```python
from build123d import *

# Parameters (mm, degrees)
SALIENTE_EXTRUIR1_DEPTH = 233
VACIADO1_T              = -2
SALIENTE_EXTRUIR2_REACH = 250.108
CROQUIS3_R              = 3.999999999999999
CROQUIS3_R_2            = 4.000000000000005
CROQUIS3_R_3            = 4.000000000000013
CROQUIS3_R_4            = 4.000000000000007
CROQUIS3_R_5            = 4.000000000000002
CROQUIS3_R_6            = 4
CROQUIS4_R              = 1.5000000000000007
CROQUIS4_R_2            = 1.4999999999999973
CROQUIS4_R_3            = 1.5000000000000042
CROQUIS4_R_4            = 1.5000000000000024
CROQUIS4_R_5            = 1.5000000000000009
CORTAR_EXTRUIR1_DEPTH   = 10
CROQUIS5_R              = 1.7500000000000002
CROQUIS5_R_2            = 1.7499999999999893
CROQUIS5_R_3            = 1.7500000000000038
CROQUIS5_R_4            = 1.749999999999997
CROQUIS5_R_5            = 1.7499999999999987
CROQUIS5_R_6            = 1.7500000000000004
CORTAR_EXTRUIR2_DEPTH   = 5
CROQUIS6_R              = 2.0000000000000036
CROQUIS6_R_2            = 1.9999999999999967
CROQUIS6_R_3            = 1.99999999999999
CROQUIS6_R_4            = 2.000000000000003
CORTAR_EXTRUIR3_DEPTH   = 1
CORTAR_EXTRUIR4_DEPTH   = 2
REDONDEO1_R             = 1


with BuildPart() as part:
    # Croquis1 → Saliente-Extruir1 (new body)
    with BuildSketch(Plane.XY):
        Polygon((82.35016819503933, 0), (82.35016819503927, 5.229344564858981), (80.29329266619476, 28.7395394398242), (78.30090327001128, 28.565227954328893), (1.9923893961834915, 21.889098059858902), (-1.33e-15, 21.7147865743636), (1.899797656141601, 0), align=None)
    extrude(amount=SALIENTE_EXTRUIR1_DEPTH)

    # Vaciado1
    vaciado1_openings = [part.faces().sort_by_distance(p)[0] for p in [
        (40.146646333, 25.227163007, 116.5),
    ]]
    offset(amount=VACIADO1_T, openings=vaciado1_openings, kind=Kind.INTERSECTION)

    # Saliente-Extruir2: up to this plane
    saliente_extruir2_end = Plane(origin=(1.899797656141601, 2, 233), z_dir=(0, 1, 0))
    # Croquis3 → Saliente-Extruir2 (add, up to the surface)
    with BuildSketch(Plane(origin=(-0.9092222397584271, 10.392457755273615, 0), x_dir=(0.9961946980917462, 0.08715574274765005, 0), z_dir=(-0.08715574274765005, 0.9961946980917462, 0)), mode=Mode.PRIVATE) as saliente_extruir2_sk1:
        with Locations((23.14256835249537, -4.200000000000009)):
            Circle(CROQUIS3_R)
    saliente_extruir2_tool1 = split(extrude(saliente_extruir2_sk1.sketch, amount=-SALIENTE_EXTRUIR2_REACH, mode=Mode.PRIVATE), bisect_by=saliente_extruir2_end, keep=Keep.BOTH, mode=Mode.PRIVATE)
    add(saliente_extruir2_tool1.solids().sort_by_distance((22.145282, 12.409465, 4.2))[0])
    # Croquis3 → Saliente-Extruir2 (add, up to the surface)
    with BuildSketch(Plane(origin=(-0.9092222397584271, 10.392457755273615, 0), x_dir=(0.9961946980917462, 0.08715574274765005, 0), z_dir=(-0.08715574274765005, 0.9961946980917462, 0)), mode=Mode.PRIVATE) as saliente_extruir2_sk2:
        with Locations(Location((61.24256835249536, -21.250000000000004, 0), (0, 0, 180))):
            Circle(CROQUIS3_R_2)
    saliente_extruir2_tool2 = split(extrude(saliente_extruir2_sk2.sketch, amount=-SALIENTE_EXTRUIR2_REACH, mode=Mode.PRIVATE), bisect_by=saliente_extruir2_end, keep=Keep.BOTH, mode=Mode.PRIVATE)
    add(saliente_extruir2_tool2.solids().sort_by_distance((60.1003, 15.730099, 21.25))[0])
    # Croquis3 → Saliente-Extruir2 (add, up to the surface)
    with BuildSketch(Plane(origin=(-0.9092222397584271, 10.392457755273615, 0), x_dir=(0.9961946980917462, 0.08715574274765005, 0), z_dir=(-0.08715574274765005, 0.9961946980917462, 0)), mode=Mode.PRIVATE) as saliente_extruir2_sk3:
        with Locations(Location((42.19256835249537, -97.45, 0), (0, 0, 180))):
            Circle(CROQUIS3_R_3)
    saliente_extruir2_tool3 = split(extrude(saliente_extruir2_sk3.sketch, amount=-SALIENTE_EXTRUIR2_REACH, mode=Mode.PRIVATE), bisect_by=saliente_extruir2_end, keep=Keep.BOTH, mode=Mode.PRIVATE)
    add(saliente_extruir2_tool3.solids().sort_by_distance((41.122791, 14.069782, 97.45))[0])
    # Croquis3 → Saliente-Extruir2 (add, up to the surface)
    with BuildSketch(Plane(origin=(-0.9092222397584271, 10.392457755273615, 0), x_dir=(0.9961946980917462, 0.08715574274765005, 0), z_dir=(-0.08715574274765005, 0.9961946980917462, 0)), mode=Mode.PRIVATE) as saliente_extruir2_sk4:
        with Locations(Location((61.24256835249536, -116.5, 0), (0, 0, 180))):
            Circle(CROQUIS3_R_4)
    saliente_extruir2_tool4 = split(extrude(saliente_extruir2_sk4.sketch, amount=-SALIENTE_EXTRUIR2_REACH, mode=Mode.PRIVATE), bisect_by=saliente_extruir2_end, keep=Keep.BOTH, mode=Mode.PRIVATE)
    add(saliente_extruir2_tool4.solids().sort_by_distance((60.1003, 15.730099, 116.5))[0])
    # Croquis3 → Saliente-Extruir2 (add, up to the surface)
    with BuildSketch(Plane(origin=(-0.9092222397584271, 10.392457755273615, 0), x_dir=(0.9961946980917462, 0.08715574274765005, 0), z_dir=(-0.08715574274765005, 0.9961946980917462, 0)), mode=Mode.PRIVATE) as saliente_extruir2_sk5:
        with Locations(Location((13.62256835249537, -128.26000000000002, 0), (0, 0, 180))):
            Circle(CROQUIS3_R_5)
    saliente_extruir2_tool5 = split(extrude(saliente_extruir2_sk5.sketch, amount=-SALIENTE_EXTRUIR2_REACH, mode=Mode.PRIVATE), bisect_by=saliente_extruir2_end, keep=Keep.BOTH, mode=Mode.PRIVATE)
    add(saliente_extruir2_tool5.solids().sort_by_distance((12.661508, 11.579743, 128.26))[0])
    # Croquis3 → Saliente-Extruir2 (add, up to the surface)
    with BuildSketch(Plane(origin=(-0.9092222397584271, 10.392457755273615, 0), x_dir=(0.9961946980917462, 0.08715574274765005, 0), z_dir=(-0.08715574274765005, 0.9961946980917462, 0)), mode=Mode.PRIVATE) as saliente_extruir2_sk6:
        with Locations((23.14256835249537, -228.8)):
            Circle(CROQUIS3_R_6)
    saliente_extruir2_tool6 = split(extrude(saliente_extruir2_sk6.sketch, amount=-SALIENTE_EXTRUIR2_REACH, mode=Mode.PRIVATE), bisect_by=saliente_extruir2_end, keep=Keep.BOTH, mode=Mode.PRIVATE)
    add(saliente_extruir2_tool6.solids().sort_by_distance((22.145282, 12.409465, 228.8))[0])
    # Croquis3 → Saliente-Extruir2 (add, up to the surface)
    with BuildSketch(Plane(origin=(-0.9092222397584271, 10.392457755273615, 0), x_dir=(0.9961946980917462, 0.08715574274765005, 0), z_dir=(-0.08715574274765005, 0.9961946980917462, 0)), mode=Mode.PRIVATE) as saliente_extruir2_sk7:
        with Locations(Location((61.24256835249536, -211.75000000000003, 0), (0, 0, 180))):
            Circle(CROQUIS3_R_4)
    saliente_extruir2_tool7 = split(extrude(saliente_extruir2_sk7.sketch, amount=-SALIENTE_EXTRUIR2_REACH, mode=Mode.PRIVATE), bisect_by=saliente_extruir2_end, keep=Keep.BOTH, mode=Mode.PRIVATE)
    add(saliente_extruir2_tool7.solids().sort_by_distance((60.1003, 15.730099, 211.75))[0])

    # Croquis4 → Cortar-Extruir1 (cut)
    with BuildSketch(Plane(origin=(-0.9092222397584271, 10.392457755273613, 0), x_dir=(0.9961946980917462, 0.08715574274765006, 0), z_dir=(-0.08715574274765006, 0.9961946980917462, 0))):
        with Locations(Location((23.142568352495374, -4.200000000000009, 0), (0, 0, 180))):
            Circle(CROQUIS4_R)
        with Locations(Location((61.24256835249536, -21.250000000000004, 0), (0, 0, 180))):
            Circle(CROQUIS4_R_2)
        with Locations(Location((42.192568352495364, -97.45, 0), (0, 0, 180))):
            Circle(CROQUIS4_R_3)
        with Locations(Location((61.24256835249536, -116.5, 0), (0, 0, 180))):
            Circle(CROQUIS4_R_2)
        with Locations(Location((13.622568352495366, -128.26000000000002, 0), (0, 0, 180))):
            Circle(CROQUIS4_R_4)
        with Locations(Location((61.24256835249536, -211.75000000000003, 0), (0, 0, 180))):
            Circle(CROQUIS4_R_2)
        with Locations(Location((23.142568352495374, -228.8, 0), (0, 0, 180))):
            Circle(CROQUIS4_R_5)
    extrude(amount=-CORTAR_EXTRUIR1_DEPTH, mode=Mode.SUBTRACT)

    # Croquis5 → Cortar-Extruir2 (cut)
    with BuildSketch(Plane(origin=(-0.9092222397584274, 10.392457755273616, 0), x_dir=(0.9961946980917462, 0.08715574274765006, 0), z_dir=(-0.08715574274765006, 0.9961946980917462, 0))):
        with Locations(Location((23.14256835249537, -4.200000000000009, 0), (0, 0, 180))):
            Circle(CROQUIS5_R)
        with Locations(Location((61.242568352495354, -21.250000000000004, 0), (0, 0, 180))):
            Circle(CROQUIS5_R_2)
        with Locations(Location((42.192568352495364, -97.45, 0), (0, 0, 180))):
            Circle(CROQUIS5_R_3)
        with Locations(Location((61.24256835249536, -116.5, 0), (0, 0, 180))):
            Circle(CROQUIS5_R_4)
        with Locations(Location((13.622568352495364, -128.26000000000002, 0), (0, 0, 180))):
            Circle(CROQUIS5_R_5)
        with Locations(Location((23.142568352495374, -228.8, 0), (0, 0, 180))):
            Circle(CROQUIS5_R_6)
        with Locations(Location((61.24256835249536, -211.75000000000003, 0), (0, 0, 180))):
            Circle(CROQUIS5_R_4)
    extrude(amount=-CORTAR_EXTRUIR2_DEPTH, mode=Mode.SUBTRACT)

    # Croquis6 → Cortar-Extruir3 (cut)
    with BuildSketch(Plane(origin=(-0.9092222397584271, 10.392457755273613, 0), x_dir=(0.9961946980917462, 0.08715574274765006, 0), z_dir=(-0.08715574274765006, 0.9961946980917462, 0))):
        with Locations(Location((13.622568352495366, -128.26000000000002, 0), (0, 0, 180))):
            Circle(CROQUIS6_R)
        with Locations(Location((23.142568352495374, -228.8, 0), (0, 0, 180))):
            Circle(CROQUIS6_R)
        with Locations(Location((61.24256835249536, -211.75000000000003, 0), (0, 0, 180))):
            Circle(CROQUIS6_R_2)
        with Locations(Location((61.242568352495354, -116.5, 0), (0, 0, 180))):
            Circle(CROQUIS6_R_3)
        with Locations(Location((42.192568352495364, -97.45, 0), (0, 0, 180))):
            Circle(CROQUIS6_R)
        with Locations(Location((61.24256835249536, -21.250000000000004, 0), (0, 0, 180))):
            Circle(CROQUIS6_R_2)
        with Locations(Location((23.14256835249537, -4.200000000000009, 0), (0, 0, 180))):
            Circle(CROQUIS6_R_4)
    extrude(amount=-CORTAR_EXTRUIR3_DEPTH, mode=Mode.SUBTRACT)

    # Croquis7 → Cortar-Extruir4 (cut)
    with BuildSketch(Plane(origin=(82.17865922472689, 7.189701065922963, 0), x_dir=(0, 0, -1), z_dir=(0.9961946980917464, 0.08715574274764931, 0))):
        Polygon((-55.83000000000002, -1.9678447444250866), (-43.830000000000005, -1.9678447444250844), (-43.83000000000001, 7.032155255574915), (-55.83000000000001, 7.032155255574913), align=None)
    extrude(amount=-CORTAR_EXTRUIR4_DEPTH, mode=Mode.SUBTRACT)

    # Redondeo1
    # the kernel refuses this fillet: 1 mm, written as the material it takes off along each edge
    with BuildSketch(Plane(origin=(82.5680575519084, 2.7388578196296147, 233), x_dir=(0, 0, -1), z_dir=(-0.08715574274764891, 0.9961946980917463, 0))) as redondeo1_piece_1:
        with BuildLine():
            CenterArc((REDONDEO1_R, REDONDEO1_R), REDONDEO1_R, 180, 90)
            Line((0, REDONDEO1_R), (0, 0))
            Line((0, 0), (REDONDEO1_R, 0))
        make_face()
    extrude(amount=28.6, mode=Mode.SUBTRACT)
    with BuildSketch(Plane(origin=(-0.21788935686912936, 24.20527331959297, 233), x_dir=(0.9961946980917461, 0.0871557427476515, 0), z_dir=(0.0871557427476515, -0.9961946980917462, 0))) as redondeo1_piece_2:
        with BuildLine():
            CenterArc((REDONDEO1_R, -REDONDEO1_R), REDONDEO1_R, 90, 90)
            Line((2.65e-15, -REDONDEO1_R), (0, 0))
            Line((0, 0), (REDONDEO1_R, 0))
        make_face()
    extrude(amount=26.79773353136612, mode=Mode.SUBTRACT)
    with BuildSketch(Plane(origin=(-0.21788935686912936, 24.20527331959297, 0), x_dir=(0.9961946980917461, 0.0871557427476515, 0), z_dir=(0.0871557427476515, -0.9961946980917462, 0))) as redondeo1_piece_3:
        with BuildLine():
            CenterArc((REDONDEO1_R, REDONDEO1_R), REDONDEO1_R, 180, 90)
            Line((2.65e-15, REDONDEO1_R), (0, 0))
            Line((0, 0), (REDONDEO1_R, 0))
        make_face()
    extrude(amount=26.79773353136612, mode=Mode.SUBTRACT)
    with BuildSketch(Plane(origin=(82.35016819503936, -2.5000000000000004, 233), x_dir=(0, 0, -1), z_dir=(-1.087e-14, 1, 0))) as redondeo1_piece_4:
        with BuildLine():
            CenterArc((REDONDEO1_R, REDONDEO1_R), REDONDEO1_R, 180, 90)
            Line((0, REDONDEO1_R), (0, 0))
            Line((0, 0), (REDONDEO1_R, 0))
        make_face()
    extrude(amount=10.229344564858982, mode=Mode.SUBTRACT)
    with BuildSketch(Plane(origin=(82.5680575519084, 2.738857819629615, 0), x_dir=(4e-17, 0, 1), z_dir=(-0.08715574274764891, 0.9961946980917463, 0))) as redondeo1_piece_5:
        with BuildLine():
            CenterArc((REDONDEO1_R, -REDONDEO1_R), REDONDEO1_R, 90, 90)
            Line((-1.5e-16, -REDONDEO1_R), (0, 0))
            Line((0, 0), (REDONDEO1_R, 0))
        make_face()
    extrude(amount=28.6, mode=Mode.SUBTRACT)
    with BuildSketch(Plane(origin=(82.35016819503936, -2.5000000000000004, 0), x_dir=(0, 0, 1), z_dir=(-1.087e-14, 1, 0))) as redondeo1_piece_6:
        with BuildLine():
            CenterArc((REDONDEO1_R, -REDONDEO1_R), REDONDEO1_R, 90, 90)
            Line((-1.1e-16, -REDONDEO1_R), (0, 0))
            Line((0, 0), (REDONDEO1_R, 0))
        make_face()
    extrude(amount=10.229344564858982, mode=Mode.SUBTRACT)


solid = part.part
```
The listing builds one solid part. Answer for the finished solid, in the listing's coordinates (mm). A direction names the side the tool comes from. Give positions to 0.01 mm unless a question says otherwise; leave off trailing zeros. Loops run counter-clockwise (first coordinate to the right, second up) from the corner with the lowest first, then second, coordinate; pieces in that order, holes last. Notation, with made-up numbers: (73.25, -14) - (115.25, -14) arc R7 ccw to (115.25, -9) - close; hole circle Ø10 at (39, -21). An arc over 180 degrees is marked (long way). Return JSON: item names as keys, results as strings. Group by question number.
1. Straight lines are drawn through the part: line 1 (Z direction, x = 11.5, y = 16); line 2 (Y direction, x = 55.5, z = 141); line 3 (Z direction, x = 13, y = 2.75). For each, find the intervals that lie inside material, in ascending order. Write a range as [from, to].
2. Determine the mould class of faces 3 (the cylindrical face through (61.72, 15.38, 210.53)), 4 (the flat face through (22.089, 12.405, 6.434)), 5 (the flat face through (82.35, 3, 115)) for opening direction Y: pulls with the +Y half, pulls with the -Y half, needs draft (parallel to the pull), parting line crosses it, or undercut.
3. Find section C-C (x = 49.5). Write down the section's boundary in (y, z), then the cut area to 3 significant figures.
4. Given pin 1 Ø1 at (y, z) = (23.5, 187) entering from -X; pin 2 Ø5 at (x, z) = (49.5, 121) entering from +Y; pin 3 Ø4 at (y, z) = (18.5, 85.5) entering from +X, each flat-ended and moving along its own axis, determine where each tip first touches the part or whether it passes through.
5. Find section A-A (z = 143.5). Write down the section's boundary in (x, y), then the cut area to 3 significant figures.
6. Find section B-B (x = 34.5). Write down the section's boundary in (y, z), then the cut area to 3 significant figures.
7. Which of the six approach directions +Z, -Z, +X, -X, +Y, -Y give full straight-line access (tool end or side, diameter ignored) to faces 1 (the flat face through (79.34, 16.69, 114.9)), 2 (the flat face through (39.41, 13.92, 95.73))?
Verdict:
{
 "1": {"line 1": "z = [0, 2], [231, 233]", "line 2": "y = [0, 2]", "line 3": "z = [0, 2], [124.28, 126.82], [129.7, 132.24], [231, 233]"},
 "2": {"face 3": "undercut", "face 4": "pulls with the +Y half", "face 5": "needs draft"},
 "3": {"outline": "(0, 0) - (26.05, 0) - (26.05, 2) - (2, 2) - (2, 231) - (26.05, 231) - (26.05, 233) - (0, 233) - close", "area": "562 mm^2"},
 "4": {"pin 1": "stops at x = 78.7", "pin 2": "stops at y = 2", "pin 3": "stops at x = 81.36"},
 "5": {"outline": "(0, 21.71) - (1.9, 0) - (82.35, 0) - (82.35, 5.23) - (80.29, 28.74) - (78.3, 28.57) - (80.35, 5.14) - (80.35, 2) - (3.73, 2) - (1.99, 21.89) - close", "area": "254 mm^2"},
 "6": {"outline": "(0, 0) - (24.73, 0) - (24.73, 2) - (2, 2) - (2, 231) - (24.73, 231) - (24.73, 233) - (0, 233) - close", "area": "557 mm^2"},
 "7": {"face 1": "none", "face 2": "+Y"}
}
